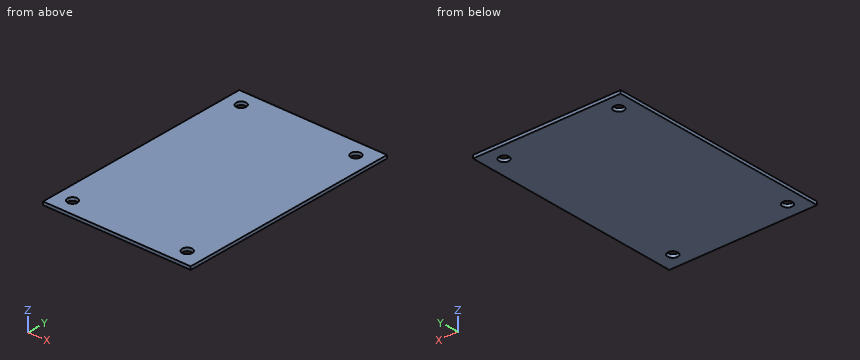
from build123d import *

# Parameters (mm, degrees)
SKETCH_1_W                  = 47
SKETCH_1_H                  = 71
EXTRUDE_1_DEPTH             = 1
SKETCH_2_R                  = 1.6
CUT_EXTRUDE_1_DEPTH         = 1
PATTERN_LINEAR_1_COUNT      = 2
PATTERN_LINEAR_1_PITCH      = 36.5
PATTERN_LINEAR_1_COUNT_DIR2 = 2
PATTERN_LINEAR_1_PITCH_DIR2 = 61


with BuildPart() as part:
    # ｽｹｯﾁ1 → ﾎﾞｽ - 押し出し1 (new body)
    with BuildSketch(Plane.XY):
        Rectangle(SKETCH_1_W, SKETCH_1_H)
    extrude(amount=EXTRUDE_1_DEPTH)

    # ｽｹｯﾁ2 → ｶｯﾄ - 押し出し1 (cut)
    with BuildSketch(Plane.XY.offset(1)):
        with Locations((-18.5, -30.5)):
            Circle(SKETCH_2_R)
    cut_extrude_1 = extrude(amount=-CUT_EXTRUDE_1_DEPTH, mode=Mode.SUBTRACT)

    # 直線ﾊﾟﾀｰﾝ1: Cut-Extrude 1 2 × 2
    with Locations(*[(i * PATTERN_LINEAR_1_PITCH, j * PATTERN_LINEAR_1_PITCH_DIR2, 0) for i in range(PATTERN_LINEAR_1_COUNT) for j in range(PATTERN_LINEAR_1_COUNT_DIR2) if (i, j) != (0, 0)]):
        add(cut_extrude_1, mode=Mode.SUBTRACT)


solid = part.part
Verification items for the finished model (mm, model axes). Round coordinates to 2 decimals unless told otherwise and drop trailing zeros. Order: outer loops, then holes, each group sorted by start corner. A loop starts at its lowest first (then second) coordinate and runs counter-clockwise, first axis right, second up. Notation, with made-up numbers: (72.5, 17.25) -> (121.5, 17.25) arc R23 cw to (121.5, 52.25) -> close; hole circle Ø4 at (12, 27). An arc over 180 degrees is marked (long way). Put each result on its own line as item: value.
1) Depth check by flat-ended pin: pin 1 (2.5 mm diameter, centred on x = -18.5, y = 30.5, fed in from +Z). Enter the tip coordinate at first touch or a pass-through.
Final values:
pin 1: passes through
2) Section check B-B (x = 18). Record the cut outline in (y, z), then the cut area to 3 significant figures.
Final values:
outline: (-35.5, 0) -> (-32.1, 0) -> (-32.1, 1) -> (-35.5, 1) -> close; (-28.9, 0) -> (28.9, 0) -> (28.9, 1) -> (-28.9, 1) -> close; (32.1, 0) -> (35.5, 0) -> (35.5, 1) -> (32.1, 1) -> close
area: 64.6 mm^2
3) Material ranges on line 1 (Y direction, x = -18.5, z = 0.85); line 2 (X direction, y = 29.5, z = 0.2), recorded low to high.
Final values:
line 1: y = -35.5 to -32.1, -28.9 to 28.9, 32.1 to 35.5
line 2: x = -23.5 to -19.75, -17.25 to 16.75, 19.25 to 23.5
4) Section check A-A (y = 30.5). Record the cut outline in (x, z).
Final values:
outline: (-23.5, 0) -> (-20.1, 0) -> (-20.1, 1) -> (-23.5, 1) -> close; (-16.9, 0) -> (16.4, 0) -> (16.4, 1) -> (-16.9, 1) -> close; (19.6, 0) -> (23.5, 0) -> (23.5, 1) -> (19.6, 1) -> close
